Autodesk Inventor part; units mm, degrees
ref_plane "YZ Plane" through (0, 0, 0) normal (1, 0, 0) x (0, 1, 0)
ref_plane "XZ Plane" through (0, 0, 0) normal (0, 1, 0) x (-1, 0, 0)
ref_plane "XY Plane" through (0, 0, 0) normal (0, 0, 1) x (1, 0, 0)
sketch "Szkic1" plane through (0, 0, 0) normal (0, 0, 1) x (1, 0, 0)
  circle A0 centre (0, 0) radius 24
  circle A1 centre (0, 0) radius 14
  dimension "d0" = 48
  dimension "d1" = 28
extrude "Wyciągnięcie proste1" add sketch "Szkic1" along normal blind 12
sketch "Szkic2" plane through (0, 0, 12) normal (0, 0, 1) x (1, 0, 0)
  circle A0 centre (0, 0) radius 19
  circle A1 centre (0, 19) radius 3
  dimension "d4" = 38
  dimension "d5" = 6
extrude "Wyciągnięcie proste2" cut sketch "Szkic2" against normal blind 12 contours A1 A0 | A0 A1 picked at (0, 17.9824) picked at (0.0843, 19.9789)
pattern_circular "Szyk kołowy1" count 6 over 360 about axis through (0, 0, 0) along (0, 0, 1) of "Wyciągnięcie proste2"
sketch "Szkic3" plane through (0, 0, 12) normal (0, 0, 1) x (1, 0, 0)
  circle A0 centre (0, 0) radius 14
  circle A1 centre (0, 0) radius 7
  dimension "d11" = 28
  dimension "d12" = 14
extrude "Wyciągnięcie proste3" add sketch "Szkic3" against normal blind 35
properties part number "Cartesian1_Z_TrapezoiadlNut" material "Brąz, miękki cynowy"
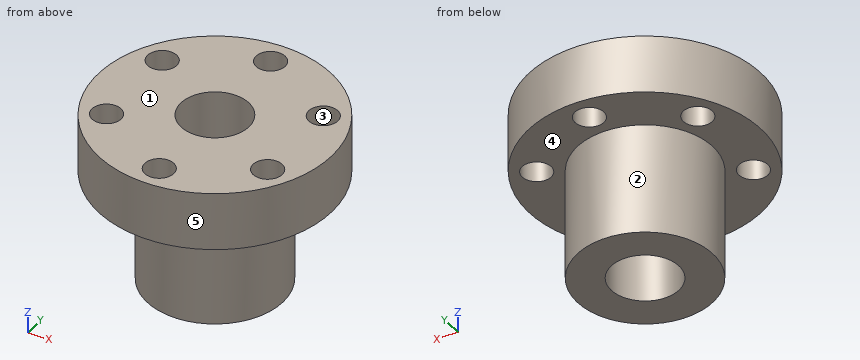
For this review, take the finished solid that the model builds, in its own axes (mm). Face numbers are marked on the shaded views. A direction names the side the tool comes from. Coordinates: 2 decimals unless noted, no trailing zeros. Loops run counter-clockwise (first coordinate to the right, second up) from the corner with the lowest first, then second, coordinate; pieces in that order, holes last.
1. Mouldability with a two-part tool opening along Y and no side actions: class the marked faces 3, 4 and 5 as +Y half, -Y half, draft (parallel to the pull), parting line (faces both ways), or undercut.
2. For the marked faces 1 and 2, list the 3-axis set-ups (+Z, -Z, +X, -X, +Y, -Y) from which the entire face can be reached by the end or side of a thin tool; tool diameter is ignored.
3. Add section B-B, the plane y = 0. Give the boundary of the cut face in (x, z), then the cut area to 3 significant figures.
4. Insertion check: P1, Ø9.5, axis at x = 0, y = -19, coming from the -Z side; P2, Ø12, axis at x = 12.5, z = -13.5, coming from the -Y side; P3, Ø1.5, axis at y = -0.5, z = -15, coming from the -X side; P4, Ø8, axis at y = 2, z = 3.5, coming from the -X side. Each pin has a flat end and moves straight along its axis. Give the tip position at first contact, or say it passes through.
5. Add section A-A, the plane x = 0. Give the boundary of the cut face in (y, z), then the cut area to 3 significant figures.
6. For line 1 (Y direction, x = 0, z = 7); line 2 (X direction, y = 10.5, z = 9); line 3 (X direction, y = 9, z = 5), list the stretches that pass through material, from the lowest coordinate up.
7. Add section C-C, the plane y = -10.5. Give the boundary of the cut face in (x, z), then the cut area to 3 significant figures.
8. Add section D-D, the plane z = -5.5. Give the boundary of the cut face in (x, y).
Result:
1. face 3: undercut
1. face 4: draft
1. face 5: parting line
2. face 1: +Z, +X, -X, +Y, -Y
2. face 2: -Z
3. outline: (-24, 0) - (-14, 0) - (-14, -23) - (-7, -23) - (-7, 12) - (-24, 12) - close; (7, -23) - (14, -23) - (14, 0) - (24, 0) - (24, 12) - (7, 12) - close
3. area: 730 mm2
4. P1: stops at z = 0
4. P2: stops at y = -12.4
4. P3: stops at x = -14
4. P4: stops at x = -24
5. outline: (-24, 0) - (-22, 0) - (-22, 12) - (-24, 12) - close; (-16, 0) - (-14, 0) - (-14, -23) - (-7, -23) - (-7, 12) - (-16, 12) - close; (7, -23) - (14, -23) - (14, 0) - (16, 0) - (16, 12) - (7, 12) - close; (22, 0) - (24, 0) - (24, 12) - (22, 12) - close
5. area: 586 mm2
6. line 1: y = -24 to -22, -16 to -7, 7 to 16, 22 to 24
6. line 2: x = -21.58 to -19.28, -13.63 to 13.63, 19.28 to 21.58
6. line 3: x = -22.25 to -19.41, -13.5 to 13.5, 19.41 to 22.25
7. outline: (-21.58, 0) - (-19.28, 0) - (-19.28, 12) - (-21.58, 12) - close; (-13.63, 0) - (-9.26, 0) - (-9.26, -23) - (9.26, -23) - (9.26, 0) - (13.63, 0) - (13.63, 12) - (-13.63, 12) - close; (19.28, 0) - (21.58, 0) - (21.58, 12) - (19.28, 12) - close
7. area: 808 mm2
8. outline: circle Ø28 at (0, 0); hole circle Ø14 at (0, 0)
